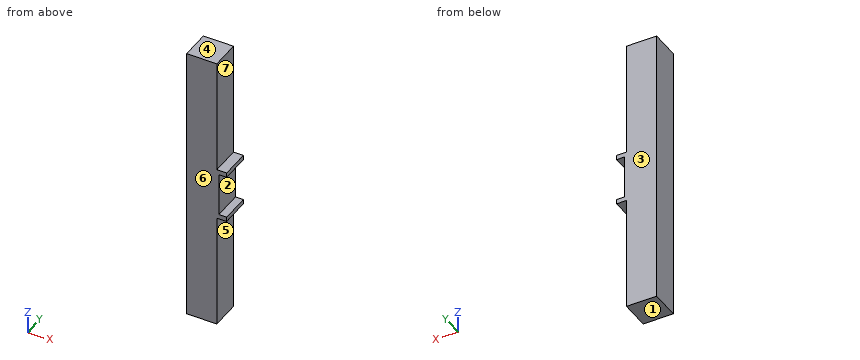
from build123d import *

# Parameters (mm, degrees)
SKETCH1_W           = 46
SKETCH1_H           = 45
BOSS_EXTRUDE1_DEPTH = 430
SKETCH2_W           = 40
SKETCH2_H           = 45
BOSS_EXTRUDE2_DEPTH = 15
SKETCH3_W           = 12
SKETCH3_H           = 66
CUT_EXTRUDE2_DEPTH  = 3434


with BuildPart() as part:
    # Sketch1 → Boss-Extrude1 (new body)
    with BuildSketch(Plane.XY):
        Rectangle(SKETCH1_W, SKETCH1_H)
    extrude(amount=BOSS_EXTRUDE1_DEPTH)

    # Sketch2 → Boss-Extrude2 (add)
    with BuildSketch(Plane(origin=(23, 0, 0), x_dir=(0, 0, -1), z_dir=(1, 0, 0))):
        with Locations((-195, 0)):
            Rectangle(SKETCH2_W, SKETCH2_H)
        with Locations((-235, 0)):
            Rectangle(SKETCH2_W, SKETCH2_H)
    extrude(amount=BOSS_EXTRUDE2_DEPTH)

    # Sketch3 → Cut-Extrude2 (cut)
    with BuildSketch(Plane(origin=(0, 22.5, 0), x_dir=(1, 0, 0), z_dir=(0, 1, 0))):
        with Locations((32, -215)):
            Rectangle(SKETCH3_W, SKETCH3_H)
    extrude(amount=-CUT_EXTRUDE2_DEPTH, mode=Mode.SUBTRACT)


solid = part.part
Here's how the part is built. I have some questions about the finished solid (model axes, mm). Face numbers are marked on the shaded views. A direction names the side the tool comes from. Round coordinates to 2 decimals unless told otherwise and drop trailing zeros. Write each loop counter-clockwise with the first axis right and the second up, starting at its lowest first coordinate (ties: lowest second). Pieces come first, ordered by that corner, then holes. Notation, with made-up numbers: (60, -22) -> (119, -22) arc R20 ccw to (119, -12) -> close; hole circle Ø9 at (75, -9). An arc over 180 degrees is marked (long way). One line per item, written item: value.
1) For the marked faces 5, 6 and 7, which set-ups out of +Z, -Z, +X, -X, +Y, -Y let a thin tool reach every point of the face, with its end or its side?
Filled sheet:
face 5: -Z, +X, +Y, -Y
face 6: +Z, -Z, +X, -X, -Y
face 7: +Z, +X, +Y, -Y
2) Suppose I cut it at A-A on x = 29.5. List the corners of the cut face in (y, z) for me, plus the area to 3 significant figures.
Filled sheet:
outline: (-22.5, 175) -> (22.5, 175) -> (22.5, 182) -> (-22.5, 182) -> close; (-22.5, 248) -> (22.5, 248) -> (22.5, 255) -> (-22.5, 255) -> close
area: 630 mm2
3) We'd pull the mould along Z, two halves only. Please class the marked faces 1, 2, 3 and 4: released by +Z, released by -Z, zero draft, split by the parting line, or undercut.
Filled sheet:
face 1: released by -Z
face 2: undercut
face 3: zero draft
face 4: released by +Z
4) I'm going to push flat-ended pins straight in: pin 1 Ø12 at (x, y) = (30, -8) entering from -Z; pin 2 Ø6 at (x, y) = (29.5, 0) entering from +Z; pin 3 Ø1.5 at (y, z) = (1, 165.5) entering from +X. Where does each tip first touch, or does it pass through?
Filled sheet:
pin 1: stops at z = 175
pin 2: stops at z = 255
pin 3: stops at x = 23
5) Suppose I cut it at D-D on z = 86. List the corners of the cut face in (x, y) for me, plus the area to 3 significant figures.
Filled sheet:
outline: (-23, -22.5) -> (23, -22.5) -> (23, 22.5) -> (-23, 22.5) -> close
area: 2,070 mm2
6) If I drill on line 1 (Z direction, x = 32, y = 13); line 2 (X direction, y = -9.5, z = 91); line 3 (Z direction, x = 25.5, y = 2), over which ranges is the centre line in solid material (lowest first)? Write a range as [from, to].
Filled sheet:
line 1: z = [175, 182], [248, 255]
line 2: x = [-23, 23]
line 3: z = [175, 255]
7) Suppose I cut it at B-B on y = -18. List the corners of the cut face in (x, z) for me.
Filled sheet:
outline: (-23, 0) -> (23, 0) -> (23, 175) -> (38, 175) -> (38, 182) -> (26, 182) -> (26, 248) -> (38, 248) -> (38, 255) -> (23, 255) -> (23, 430) -> (-23, 430) -> close
8) Suppose I cut it at C-C on z = 195.5. List the corners of the cut face in (x, y) for me.
Filled sheet:
outline: (-23, -22.5) -> (26, -22.5) -> (26, 22.5) -> (-23, 22.5) -> close
